For this review, take the finished solid that the model builds, in its own axes (mm). Face numbers are marked on the shaded views. A direction names the side the tool comes from. Coordinates: 2 decimals unless noted, no trailing zeros. Write each loop counter-clockwise with the first axis right and the second up, starting at its lowest first coordinate (ties: lowest second). Pieces come first, ordered by that corner, then holes. Notation, with made-up numbers: M 76,-16 L 94,-16 A4 cw 94,-10 Z; hole C -23,-16 d4. An arc over 180 degrees is marked long. Return JSON: item names as keys, results as strings.
```python
from build123d import *

# Parameters (mm, degrees)
CUT_EXTRUDE1_REACH = 89.396
SKETCH2_R          = 6
CIRPATTERN1_COUNT  = 6
FILLET1_R          = 2
FILLET2_R          = 1
CHAMFER1_SIZE      = 1
CHAMFER2_SIZE      = 2


with BuildPart() as part:
    # Sketch1 → Revolve1 (revolve)
    with BuildSketch(Plane(origin=(0, 0, 0), x_dir=(0, 0, -1), z_dir=(1, 0, 0)), mode=Mode.PRIVATE) as revolve1_sk:
        Polygon((-11.208917924, 22), (-11.208917924, 59), (5.791082076, 59), (5.791082076, 27), (31.791082076, 27), (31.791082076, 12), (-7.208917924, 12), (-7.208917924, 17), (-14.208917924, 17), (-14.208917924, 22), align=None)
    revolve(revolve1_sk.sketch.rotate(Axis((0, 0, 9.001223373), (0, 0, -1)), 90), axis=Axis((0, 0, 9.001223373), (0, 0, -1)))

    # Sketch2 → Cut-Extrude1 (cut, up to next)
    with BuildSketch(Plane(origin=(0, 0, -5.791082076), x_dir=(-1, 0, 0), z_dir=(0, 0, -1)), mode=Mode.PRIVATE) as cut_extrude1_sk1:
        with Locations((0, 44)):
            Circle(SKETCH2_R)
    cut_extrude1_tool1 = extrude(cut_extrude1_sk1.sketch, amount=-CUT_EXTRUDE1_REACH, mode=Mode.PRIVATE) & part.part
    cut_extrude1 = cut_extrude1_tool1.solids().sort_by_distance((0, 44, -5.791082))[0]
    add(cut_extrude1, mode=Mode.SUBTRACT)

    # CirPattern1: Cut-Extrude1 ×6 about axis
    cirpattern1_axis = Axis((0, 0, 0), (0, 0, 1))
    for i in range(1, CIRPATTERN1_COUNT):
        add(cut_extrude1.rotate(cirpattern1_axis, i * 360 / CIRPATTERN1_COUNT), mode=Mode.SUBTRACT)

    # Fillet1
    fillet1_edges = [part.edges().sort_by_distance(p)[0] for p in [
        (-27, 0, -5.791082076),
    ]]
    fillet(fillet1_edges, radius=FILLET1_R)

    # Fillet2
    fillet2_edges = [part.edges().sort_by_distance(p)[0] for p in [
        (-17, 0, 7.208917924),
    ]]
    fillet(fillet2_edges, radius=FILLET2_R)

    # Chamfer1
    chamfer1_edges = [part.edges().sort_by_distance(p)[0] for p in [
        (-12, 0, -31.791082076),
        (-27, 0, -31.791082076),
    ]]
    chamfer(chamfer1_edges, length=CHAMFER1_SIZE)

    # Chamfer2
    chamfer2_edges = [part.edges().sort_by_distance(p)[0] for p in [
        (-59, 0, -5.791082076),
    ]]
    chamfer(chamfer2_edges, length=CHAMFER2_SIZE)


solid = part.part
```
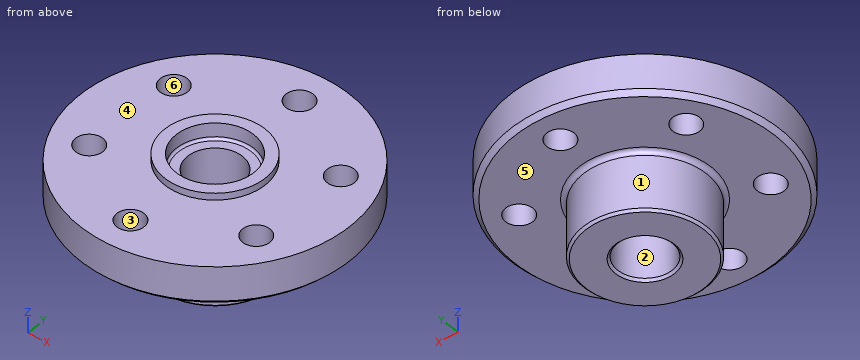
1. Clearance check with flat-ended pins moving along their axes: pin 1 Ø8 at (x, z) = (-9, 1.5) entering from +Y; pin 2 Ø5 at (x, y) = (34.5, 11.5) entering from +Z; pin 3 Ø5 at (x, z) = (-12, -24.5) entering from +Y; pin 4 Ø11 at (x, y) = (0, -44) entering from -Z. State where each tip first meets the part, or that it passes through.
Checks:
{"pin 1": "y = 58.79", "pin 2": "z = 11.21", "pin 3": "y = 25.27", "pin 4": "through"}
2. We need section C-C (x = 0). Give the number of separate pieces and of enclosed holes in the cut face, plus the area to 3 significant figures.
Checks:
{"separate pieces": "4", "enclosed holes": "0", "area": "1,960 mm2"}
3. For the marked faces 5 and 6, list the 3-axis set-ups (+Z, -Z, +X, -X, +Y, -Y) from which the entire face can be reached by the end or side of a thin tool; tool diameter is ignored.
Checks:
{"face 5": "-Z", "face 6": "+Z, -Z"}
4. Draft analysis for pull direction Y (two halves, no side actions). For the marked faces 1, 2, 3 and 4, state which applies: +Y half, -Y half, draft (parallel to the pull), parting line (faces both ways), or undercut.
Checks:
{"face 1": "parting line", "face 2": "undercut", "face 3": "undercut", "face 4": "draft"}
5. We need section B-B (z = -22). State the section outline as (x, y) points.
Checks:
{"outline": "C 0,0 d54; hole C 0,0 d24"}
6. Wall thickness on L1, parallel to Y at x = 0, z = 0.25; L2, parallel to Y at x = 0, z = 10.9; L3, parallel to Y at x = -42, z = -1: over which ranges is each line inside the solid? List them lowest first. Write a range as from..to.
Checks:
{"L1": "-59..-50, -38..-12, 12..38, 50..59", "L2": "-59..-50, -38..-17, 17..38, 50..59", "L3": "-41.44..-26.56, -17.44..17.44, 26.56..41.44"}
